Could you check a few things on this model? Use its own coordinates, in mm. Face numbers are marked on the shaded views. Round coordinates to 2 decimals unless told otherwise and drop trailing zeros. Loops run counter-clockwise (first coordinate to the right, second up) from the corner with the lowest first, then second, coordinate; pieces in that order, holes last. Notation, with made-up numbers: M 43,9 L 59,9 A34 cw 59,46 Z; hole C -31.75,80.5 d7. An arc over 180 degrees is marked long. Return JSON: item names as keys, results as strings. Group by question number.
```python
from build123d import *

# Parameters (mm, degrees)
EXTRUDE_1_DEPTH     = 10
SKETCH_2_R          = 7
CUT_EXTRUDE_1_DEPTH = 10


with BuildPart() as part:
    # 草图1 → 凸台-拉伸1 (new body)
    with BuildSketch(Plane.XY):
        with BuildLine():
            Line((-20, 0), (20, 0))
            Line((20, 0), (12.235428647, 28.977774789))
            ThreePointArc((12.235428647, 28.977774789), (0, 38.366349399), (-12.235428647, 28.977774789))
            Line((-12.235428647, 28.977774789), (-20, 0))
        make_face()
    extrude(amount=EXTRUDE_1_DEPTH)

    # 草图2 → 切除-拉伸1 (cut)
    with BuildSketch(Plane.XY):
        with Locations((0, 25.699301564)):
            Circle(SKETCH_2_R)
    extrude(amount=CUT_EXTRUDE_1_DEPTH, mode=Mode.SUBTRACT)


solid = part.part
```
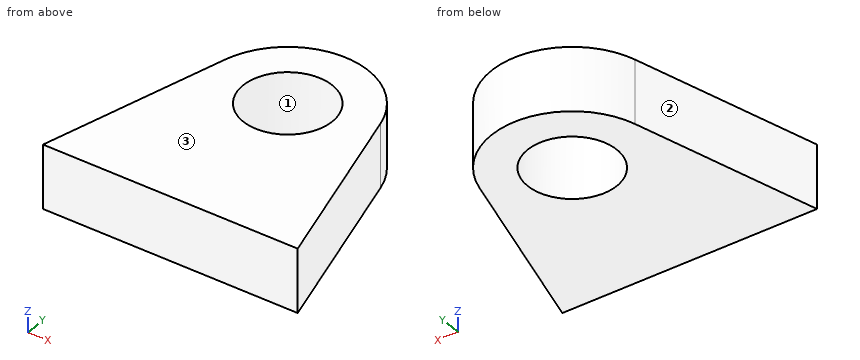
1. If we section it at A-A, the plane x = 0: Please give me the cut outline in (y, z).
2. If we section it at C-C, the plane z = 8.75: Please give me the cut outline in (x, y).
3. If we section it at D-D, the plane y = 13.5: Please give me the cut outline in (x, z).
4. I'm going to push flat-ended pins straight in: pin 1 Ø5 at (y, z) = (31.5, 3.5) entering from -X; pin 2 Ø5 at (y, z) = (8.5, 1) entering from +X; pin 3 Ø2 at (y, z) = (12, 6) entering from -X. Where does each tip first touch, or does it pass through?
5. If we section it at B-B, the plane y = 21: Please give me the cut outline in (x, z).
6. I need wall thicknesses on probe 1 along Y at (x, z) = (-5.5, 1.5); probe 2 along X at (y, z) = (31, 8.5); probe 3 along X at (y, z) = (32, 1.5). Which ranges of each line are inside material? Lowest first, please.
7. We'd pull the mould along Y, two halves only. Please class the marked faces 1, 2 and 3: +Y half, -Y half, draft (parallel to the pull), parting line (faces both ways), or undercut.
Geometry results:
{
 "1": {"outline": "M 0,0 L 18.7,0 L 18.7,10 L 0,10 Z; M 32.7,0 L 38.37,0 L 38.37,10 L 32.7,10 Z"},
 "2": {"outline": "M -20,0 L 20,0 L 12.24,28.98 A12.67 ccw -12.24,28.98 Z; hole C 0,25.7 d14"},
 "3": {"outline": "M -16.38,0 L 16.38,0 L 16.38,10 L -16.38,10 Z"},
 "4": {"pin 1": "x = -12.23", "pin 2": "x = 18.39", "pin 3": "x = -17.05"},
 "5": {"outline": "M -14.37,0 L -5.19,0 L -5.19,10 L -14.37,10 Z; M 5.19,0 L 14.37,0 L 14.37,10 L 5.19,10 Z"},
 "6": {"probe 1": "0 to 21.37, 30.03 to 37.11", "probe 2": "-11.5 to -4.57, 4.57 to 11.5", "probe 3": "-10.99 to -3.05, 3.05 to 10.99"},
 "7": {"face 1": "undercut", "face 2": "+Y half", "face 3": "draft"}
}
